Input: part model. Units: mm. Frame: model coordinates. Coordinates: 2 decimals unless noted, no trailing zeros. Order: outer loops, then holes, each group sorted by start corner. A loop starts at its lowest first (then second) coordinate and runs counter-clockwise, first axis right, second up.
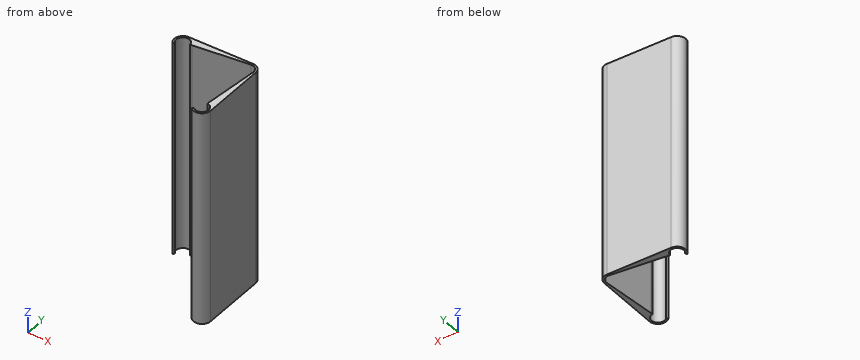
Autodesk Inventor part; units mm, degrees
ref_plane "YZ Plane" through (0, 0, 0) normal (1, 0, 0) x (0, 1, 0)
ref_plane "XZ Plane" through (0, 0, 0) normal (0, 1, 0) x (-1, 0, 0)
ref_plane "XY Plane" through (0, 0, 0) normal (0, 0, 1) x (1, 0, 0)
sketch "Sketch2" plane through (0, 0, 0) normal (0, 0, 1) x (1, 0, 0)
  arc A0 (-11.9166, 15.3203) -> (-17.192, 12.808) centre (-15, 15) ccw
  arc A1 (18.0834, 14.6797) -> (14.6797, 18.0834) centre (15, 15) ccw
  arc A2 (12.808, -17.192) -> (15.3203, -11.9166) centre (15, -15) ccw
  arc A3 (12.1716, -17.8284) -> (15.4133, -11.0214) centre (15, -15) ccw
  line L0 (-15, 19) -> (15, 19)
  line L1 (19, 15) -> (19, -15)
  line L2 (-15, 15) -> (-17.8284, 12.1716)
  line L3 (-15, 15) -> (-11, 15) construction
  line L4 (-15, 15) -> (14.6797, 18.0834)
  line L5 (15, -15) -> (18.0834, 14.6797)
  line L6 (15, -15) -> (12.1716, -17.8284)
  arc A4 (-11.0214, 15.4133) -> (-17.8284, 12.1716) centre (-15, 15) ccw
  arc A5 (19, 15) -> (15, 19) centre (15, 15) ccw
  point P0 (0, 0)
  dimension "d18" = 6.2
  dimension "d19" = 6.2
  dimension "d22" = 8
  dimension "d24" = 135
extrude "Extrusion2" add sketch "Sketch2" along normal blind 100 contours A0 L2 A4 L4 | A4 L0 A5 L1 A3 L5 A1 L4 | A3 L6 A2 L5
properties part number "Cage30mm-2sides-L100mm"
Item 1: Cut plane C-C on x = 7. Return loops of the section in (y, z), then the cut area to 3 significant figures.
Response values:
outline: (17.29, 0) - (19, 0) - (19, 100) - (17.29, 100) - close
area: 171 mm2
Item 2: Cut plane B-B on y = 3. Return loops of the section in (x, z).
Response values:
outline: (16.87, 0) - (19, 0) - (19, 100) - (16.87, 100) - close
Item 3: Cut plane A-A on z = 62. Return loops of the section in (x, y).
Response values:
outline: (-17.83, 12.17) - (-17.19, 12.81) arc R3.1 cw (long way) to (-11.92, 15.32) - (14.68, 18.08) arc R3.1 cw to (18.08, 14.68) - (15.32, -11.92) arc R3.1 cw (long way) to (12.81, -17.19) - (12.17, -17.83) arc R4 ccw to (19, -15) - (19, 15) arc R4 ccw to (15, 19) - (-15, 19) arc R4 ccw to start
Item 4: Ray query, probe 1 along Y at (x, z) = (13, 61); probe 2 along X at (y, z) = (14, 67.5); probe 3 along Y at (x, z) = (-15, 85). Return the intervals inside material, ascending.
Response values:
probe 1: y = -18.46 to -17.37, 17.91 to 19
probe 2: x = -18.87 to -17.93, 18.01 to 19
probe 3: y = 18.1 to 19
Item 5: Pin query (flat end, axial travel): pin 1 Ø1.5 at (y, z) = (-6, 54.5) entering from -X; pin 2 Ø4 at (x, z) = (7.5, 86.5) entering from -Y. Return the tip coordinate at first contact, or that it passes through.
Response values:
pin 1: stops at x = 15.86
pin 2: stops at y = 17.13
